Source: CAD feature listing. Evaluate the final solid. Frame: model axes, mm. Face numbers are marked on the shaded views. A direction names the side the tool comes from. Give positions to 0.01 mm unless a question says otherwise; leave off trailing zeros. Loops run counter-clockwise (first coordinate to the right, second up) from the corner with the lowest first, then second, coordinate; pieces in that order, holes last.
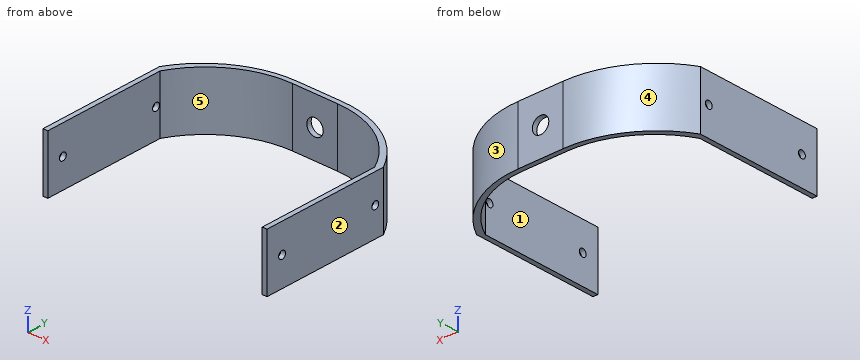
Autodesk Inventor part; units mm, degrees
ref_plane "YZ Plane" through (0, 0, 0) normal (1, 0, 0) x (0, 1, 0)
ref_plane "XZ Plane" through (0, 0, 0) normal (0, 1, 0) x (-1, 0, 0)
ref_plane "XY Plane" through (0, 0, 0) normal (0, 0, 1) x (1, 0, 0)
sketch "Sketch1" plane through (0, 0, 0) normal (0, 0, 1) x (1, 0, 0)
  line L0 (0, 0) -> (3.2, 0)
  line L1 (3.2, 0) -> (3.2, 82)
  line L2 (0, 0) -> (0, 85)
  line L3 (146.8, 82) -> (146.8, 0)
  line L4 (146.8, 0) -> (150, 0)
  line L5 (150, 0) -> (150, 85)
  arc A0 (60, 116.8) -> (3.2, 82) centre (60, 53.046) ccw
  line L6 (60, 116.8) -> (90, 116.8)
  arc A1 (146.8, 82) -> (90, 116.8) centre (90, 53.046) ccw
  arc A2 (60, 120) -> (0, 85) centre (60, 51.0714) ccw
  line L7 (60, 120) -> (90, 120)
  arc A3 (150, 85) -> (90, 120) centre (90, 51.0714) ccw
  point P0 (75, 120)
  point P1 (75, 116.8)
  dimension "d0" = 3.2
  dimension "d1" = 3.2
  dimension "d2" = 3.2
  dimension "d3" = 150
  dimension "d4" = 120
  dimension "d5" = 30
  dimension "d12" = 85
  dimension "d13" = 75
  dimension "d14" = 3
  dimension "d15" = 30
  dimension "d16" = 85
  dimension "d17" = 8
extrude "Extrusion1" add sketch "Sketch1" along normal blind 38.2
sketch "Sketch2" plane through (150, 0, 0) normal (1, 0, 0) x (0, 0, -1)
  circle A0 centre (-19.1, 11) radius 2.5
  circle A1 centre (-19.1, 79) radius 2.5
  line L0 (0, 0) -> (0, 85)
  line L1 (0, 0) -> (-38.2, 0)
  dimension "d8" = 19.1
  dimension "d9" = 5
  dimension "d10" = 68
  dimension "d11" = 11
extrude "Extrusion2" cut sketch "Sketch2" against normal through all
sketch "Sketch3" plane through (60, 120, 0) normal (0, 1, 0) x (1, 0, 0)
  circle A0 centre (15, -19.1) radius 5.5
  line L0 (-60, 0) -> (-60, -38.2)
  line L1 (30, 0) -> (0, 0)
  dimension "d20" = 11
  dimension "d21" = 75
  dimension "d22" = 19.1
extrude "Extrusion3" cut sketch "Sketch3" against normal blind 10
properties part number "shin_bracket"
(1) Section B-B, the plane x = 75. Return the cut outline in (y, z), then the cut area to 3 significant figures.
A:
outline: (116.8, 0) - (120, 0) - (120, 13.6) - (116.8, 13.6) - close; (116.8, 24.6) - (120, 24.6) - (120, 38.2) - (116.8, 38.2) - close
area: 87.0 mm2
(2) Reachability of the marked faces 1 and 2 from +Z, -Z, +X, -X, +Y, -Y: full face, straight path, thin tool, end or side. Return the list, or none.
A:
face 1: +Z, -Z, -Y
face 2: +Z, -Z, +X, +Y, -Y
(3) First-contact query: pin 1 (12 mm diameter, centred on x = 20.5, z = 5.5, fed in from -Y); pin 2 (4.5 mm diameter, centred on y = 79, z = 19.1, fed in from +X); pin 3 (12 mm diameter, centred on x = 115.5, z = 9, fed in from +Y). Flat tips, straight axial feed; report the tip coordinate or a pass-through.
A:
pin 1: stops at y = 97.7
pin 2: passes through
pin 3: stops at y = 117.18
(4) Section C-C, the plane z = 19.1. Count the separate pieces of the cut face and the enclosed holes in it, then the cut area to 3 significant figures.
A:
separate pieces: 6
enclosed holes: 0
area: 1,040 mm2
(5) Ray query, line 1 along X through (y, z) = (26, 34); line 2 along Y through (x, z) = (149.05, 19.1); line 3 along Y through (x, z) = (1, 19). Return the intervals inside material, ascending.
A:
line 1: x = 0 to 3.2, 146.8 to 150
line 2: y = 0 to 8.5, 13.5 to 76.5, 81.5 to 86.63
line 3: y = 0 to 8.5, 13.5 to 76.5, 81.5 to 86.71
(6) Mould query, pull axis X, two halves, no side actions, for the marked faces 3, 4 and 5. Classes: pulls with the +X half, pulls with the -X half, needs draft (parallel to the pull), parting line crosses it, or undercut.
A:
face 3: pulls with the +X half
face 4: pulls with the -X half
face 5: undercut
(7) Section D-D, the plane y = 23. Return the cut outline in (x, z).
A:
outline: (0, 0) - (3.2, 0) - (3.2, 38.2) - (0, 38.2) - close; (146.8, 0) - (150, 0) - (150, 38.2) - (146.8, 38.2) - close
(8) Section A-A, the plane y = 11. Return the cut outline in (x, z), then the cut area to 3 significant figures.
A:
outline: (0, 0) - (3.2, 0) - (3.2, 16.6) - (0, 16.6) - close; (0, 21.6) - (3.2, 21.6) - (3.2, 38.2) - (0, 38.2) - close; (146.8, 0) - (150, 0) - (150, 16.6) - (146.8, 16.6) - close; (146.8, 21.6) - (150, 21.6) - (150, 38.2) - (146.8, 38.2) - close
area: 212 mm2
